Design review of the part built by this model. Coordinates are the model's own, in mm. Give positions to 0.01 mm unless a question says otherwise; leave off trailing zeros. Loops run counter-clockwise (first coordinate to the right, second up) from the corner with the lowest first, then second, coordinate; pieces in that order, holes last. Notation, with made-up numbers: (29.5, 65.5) -> (40.5, 65.5) arc R23 cw to (40.5, 88.5) -> close; hole circle Ø6 at (10.5, 72). An arc over 180 degrees is marked (long way). Answer as CSV lines item,"result".
Autodesk Inventor part; units mm, degrees
ref_plane "Cross Section Plane" through (20.0445, -42.3924, 0) normal (1, 0.004, 0) x (0, 0, 1)
ref_plane "Work Plane2" through (20, -31.2516, 0) normal (-1, 0, 0) x (0, 0, 1)
ref_plane "Work Plane3" through (270.5, -30.2516, 0) normal (-0.984, 0.1784, 0) x (0, 0, 1)
sketch "Sketch Path" plane through (0, 0, 0) normal (0, 0, 1) x (1, 0, 0)
  arc A0 (19.9555, -20.1108) -> (20.0445, -42.3924) centre (20, -31.2516) ccw
  arc A1 (270.5445, -41.3924) -> (270.4555, -19.1108) centre (270.5, -30.2516) ccw
  line L0 (270.5445, -41.3924) -> (20.0445, -42.3924)
  line L1 (19.9555, -20.1108) -> (270.4555, -19.1108)
  point P0 (10.0164, 35.326)
  point P1 (9.9836, 27.3683)
  point P2 (270.4836, 26.296)
  point P3 (270.5164, 34.2537)
  point P4 (9.9836, -27.3683)
  point P5 (10.0164, -35.326)
  point P6 (270.5164, -34.2537)
  point P7 (270.4836, -26.296)
  point P8 (20.2708, -20.2096)
  point P9 (20.3662, -42.482)
  point P10 (270.6308, -34.2516)
  point P11 (270.5967, -26.2972)
  point P12 (19.9523, -20.2064)
  point P13 (20.0477, -42.4879)
  point P14 (270.5477, -41.4156)
  point P15 (270.4523, -19.1341)
ref_plane "Cross Section Plane" through (20.0445, -42.3924, 0) normal (1, 0.004, 0) x (0, 0, 1)
ref_plane "Work Plane2" through (20, -31.2516, 0) normal (-1, 0, 0) x (0, 0, 1)
ref_plane "Work Plane3" through (270.5, -30.2516, 0) normal (-0.984, 0.1784, 0) x (0, 0, 1)
ref_plane "Work Plane4" through (20, -42.488, 0) normal (0, 0, -1) x (-1, 0, 0)
sketch3d "Sketch3"
feature "iSBeltToothT:1" [suppressed]
pattern_linear "Rectangular Pattern1" [suppressed]
sketch "Cross Section" plane through (20.0445, -42.3924, 0) normal (1, 0.004, 0) x (0, 0, 1)
  line L0 (-3, 0.3) -> (3, 0.3)
  line L1 (3, 0.3) -> (3, -0.3)
  line L2 (3, -0.3) -> (-3, -0.3)
  line L3 (-3, -0.3) -> (-3, 0.3)
  line L4 (-3, 0) -> (3, 0) construction
  point P0 (0, 0)
  point P1 (0, 0)
  dimension "d0" = 6
  dimension "d4" = 0.3
  dimension "d5" = 0.3
sweep "Belt" add profiles "Cross Section" path "Sketch Path"
fillet "Fillet1" [suppressed]
equation "\"d0\" = da_B"
equation "\"d4\" = da_a"
equation "\"d5\" = da_a2"
equation "\"d21\" = d13"
equation "\"d20\" = da_pb"
equation "\"da_B\" = 6"
equation "\"da_pb\" = 2.5"
equation "\"da_L\" = 571.00399"
equation "\"da_a\" = 0.3"
equation "\"da_S\" = 1.5"
equation "\"da_Beta\" = 20deg"
equation "\"da_Ht\" = 0.7"
equation "\"da_H\" = 1.3"
equation "\"da_a2\" = 0.3"
properties part number "Synchronous Belt" material "Rubber"
Q1. We need section C-C, the plane x = 152. State the section outline as (y, z) points, and give its area (3 significant figures).
Filled sheet:
outline,"(-42.17, -3) -> (-41.57, -3) -> (-41.57, 3) -> (-42.17, 3) -> close; (-19.88, -3) -> (-19.28, -3) -> (-19.28, 3) -> (-19.88, 3) -> close"
area,"7.20 mm^2"
Q2. The part is to be moulded in two halves that separate along X. For faces 1 (the cylindrical face through (9.16, -31.06, 0.04)), 2 (the flat face through (146, -42, 3)), 3 (the cylindrical face through (281.34, -30.45, 0.04)), say which applies: pulls with the +X half, pulls with the -X half, needs draft (parallel to the pull), parting line crosses it, or undercut.
Filled sheet:
face 1,"undercut"
face 2,"needs draft"
face 3,"undercut"
Q3. To check wall thickness, follow probe 1 along Y at (x, z) = (22, -0.2); probe 2 along X at (y, z) = (-31.25, 1.8); probe 3 along X at (y, z) = (-23.75, -0.25). State the ranges of each line that lie inside material, in increasing order. Write a range as from..to.
Filled sheet:
probe 1,"y = -42.68..-42.08, -20.4..-19.8"
probe 2,"x = 8.56..9.16, 281.29..281.9"
probe 3,"x = 11.36..12.17, 279.17..279.91"
Q4. We need section B-B, the plane y = -30.5. State the section outline as (x, z) points, and give its area (3 significant figures).
Filled sheet:
outline,"(8.58, -3) -> (9.19, -3) -> (9.19, 3) -> (8.58, 3) -> close; (281.34, -3) -> (281.94, -3) -> (281.94, 3) -> (281.34, 3) -> close"
area,"7.21 mm^2"
Q5. Clearance check with a flat-ended pin moving along its axis: pin 1 Ø2 at (x, z) = (188, 2) entering from +Y. State where the tip first meets the part, or that it passes through.
Filled sheet:
pin 1,"stops at y = -19.14"
Q6. We need section A-A, the plane z = 1.55. State the section outline as (x, y) points.
Filled sheet:
outline,"(19.95, -19.81) arc R11.44 ccw to (20.05, -42.69) -> (270.55, -41.69) arc R11.44 ccw to (270.45, -18.81) -> close; hole (19.96, -20.41) arc R10.84 ccw to (20.04, -42.09) -> (270.54, -41.09) arc R10.84 ccw to (270.46, -19.41) -> close"
